Source: CAD feature listing. Evaluate the final solid. Frame: model axes, mm. Give positions to 0.01 mm unless a question says otherwise; leave off trailing zeros. Order: outer loops, then holes, each group sorted by start corner. A loop starts at its lowest first (then second) coordinate and runs counter-clockwise, first axis right, second up.
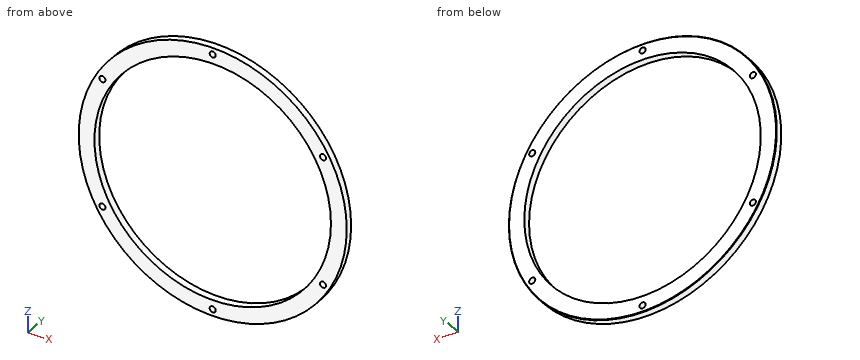
from build123d import *

# Parameters (mm, degrees)
SKETCH_1_R      = 55.25
SKETCH_1_R_2    = 48.75
EXTRUDE_1_DEPTH = 3
M3X0_5_1_D      = 2.5
CHAMFER_1_SIZE  = 0.2


with BuildPart() as part:
    # 草图1 → 凸台-拉伸1 (new body)
    with BuildSketch(Plane(origin=(0, 0, 0), x_dir=(1, 0, 0), z_dir=(0, 1, 0))):
        Circle(SKETCH_1_R)
        Circle(SKETCH_1_R_2, mode=Mode.SUBTRACT)
    extrude(amount=EXTRUDE_1_DEPTH)

    # M3x0.5 螺纹孔1 (through all)
    with Locations(Plane(origin=(0, 3, -52.525), x_dir=(0, 0, 1), z_dir=(0, 1, 0))):
        with Locations((0, 0), (26.2625, 45.487984334), (78.7875, 45.487984334), (105.05, 0), (78.7875, -45.487984334), (26.2625, -45.487984334)):
            Hole(M3X0_5_1_D / 2)

    # 倒角1
    chamfer_1_edges = [part.edges().sort_by_distance(p)[0] for p in [
        (-55.25, 3, 0),
    ]]
    chamfer(chamfer_1_edges, length=CHAMFER_1_SIZE)


solid = part.part
(1) Pin query (flat end, axial travel): pin 1 Ø1.5 at (y, z) = (2.5, -33) entering from -X; pin 2 Ø2 at (x, z) = (-45.49, -26.26) entering from -Y. Return the tip coordinate at first contact, or that it passes through.
(2) Section A-A, the plane z = 0. Return loops of the section in (x, y).
(3) Line query: line 1 along X through (y, z) = (1.9, 0); line 2 along Z through (x, y) = (1.5, 1.9); line 3 along X through (y, z) = (2.8, -25.5). Output: solid intervals per line, ascending.
(4) Section B-B, the plane y = 1.55. Count the separate pieces of the cut face and the enclosed holes in it, plus the area to 3 significant figures.
Checks:
1. pin 1: stops at x = -44.86
1. pin 2: passes through
2. outline: (-55.25, 0) - (-48.75, 0) - (-48.75, 3) - (-55.05, 3) - (-55.25, 2.8) - close; (48.75, 0) - (55.25, 0) - (55.25, 2.8) - (55.05, 3) - (48.75, 3) - close
3. line 1: x = -55.25 to -48.75, 48.75 to 55.25
3. line 2: z = -55.23 to -48.73, 48.73 to 55.23
3. line 3: x = -49.01 to -46.48, -44.5 to -41.55, 41.55 to 44.5, 46.48 to 49.01
4. separate pieces: 1
4. enclosed holes: 7
4. area: 2,090 mm2
